Read the model definition and answer for the solid it produces. Units are mm, in the model's axes. Face numbers are marked on the shaded views. Coordinates: 2 decimals unless noted, no trailing zeros. Write each loop counter-clockwise with the first axis right and the second up, starting at its lowest first coordinate (ties: lowest second). Pieces come first, ordered by that corner, then holes. Notation, with made-up numbers: (-3, 87) -> (16, 87) arc R16 cw to (16, 102) -> close; hole circle Ø8 at (41, 26.5). An arc over 180 degrees is marked (long way). One line per item, written item: value. Start each with the question number.
1. Find section A-A, the plane x = 0. Write down the section's boundary in (y, z) (1 decimal).
2. Find section C-C, the plane x = -6.5. Write down the section's boundary in (y, z).
3. Find section D-D, the plane z = 12. Write down the section's boundary in (x, y) (3 decimals), and give its area (3 significant figures).
4. Consider line 1 along Z through (x, y) = (15, 0); line 2 along Y through (x, z) = (0, 26) (3 decimals); line 3 along X through (y, z) = (0.5, 23.5). Determine where each line is inside the solid, lowest interval first.
5. Given P1, Ø3, axis at x = -7.5, y = 7, coming from the -Z side; P2, Ø1.5, axis at y = -7, z = 28.5, coming from the +X side; P3, Ø8, axis at x = 10, z = 29.5, coming from the +Y side; P4, Ø6, axis at x = -6.5, z = 23.5, coming from the +Y side, each flat-ended and moving along its own axis, determine where each tip first touches the part or whether it passes through.
6. For a pull along Z with two mould halves and no side action, classify the marked faces 1, 2 and 3 as pulls with the +Z half, pulls with the -Z half, needs draft (parallel to the pull), parting line crosses it, or undercut.
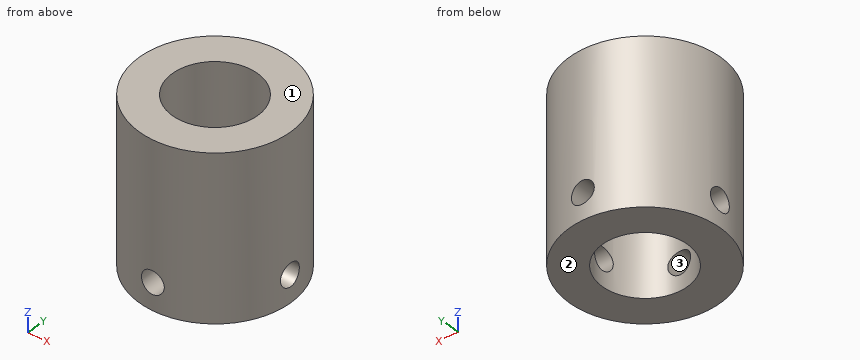
```python
from build123d import *

# Parameters (mm, degrees)
SKETCH1_R           = 16.891
SKETCH1_R_2         = 9.525
BOSS_EXTRUDE1_DEPTH = 36.5125
SKETCH2_R           = 2.54
CUT_EXTRUDE1_DEPTH  = 36.5125
CIRPATTERN1_COUNT   = 4


with BuildPart() as part:
    # Sketch1 → Boss-Extrude1 (new body)
    with BuildSketch(Plane.XY):
        Circle(SKETCH1_R)
        Circle(SKETCH1_R_2, mode=Mode.SUBTRACT)
    extrude(amount=BOSS_EXTRUDE1_DEPTH)

    # Sketch2 → Cut-Extrude1 (cut)
    with BuildSketch(Plane(origin=(16.891, 0, 0), x_dir=(0, 0, -1), z_dir=(1, 0, 0))):
        with Locations((-5.99948, 0)):
            Circle(SKETCH2_R)
    cut_extrude1 = extrude(amount=-CUT_EXTRUDE1_DEPTH, mode=Mode.SUBTRACT)

    # CirPattern1: Cut-Extrude1 ×4 about axis
    cirpattern1_axis = Axis((0, 0, 36.5125), (0, 0, -1))
    for i in range(1, CIRPATTERN1_COUNT):
        add(cut_extrude1.rotate(cirpattern1_axis, i * 360 / CIRPATTERN1_COUNT), mode=Mode.SUBTRACT)


solid = part.part
```
Answer block:
1. outline: (-16.9, 0) -> (-9.5, 0) -> (-9.5, 3.5) -> (-16.9, 3.5) -> close; (-16.9, 8.5) -> (-9.5, 8.5) -> (-9.5, 36.5) -> (-16.9, 36.5) -> close; (9.5, 0) -> (16.9, 0) -> (16.9, 3.5) -> (9.5, 3.5) -> close; (9.5, 8.5) -> (16.9, 8.5) -> (16.9, 36.5) -> (9.5, 36.5) -> close
2. outline: (-15.59, 0) -> (-6.96, 0) -> (-6.96, 36.51) -> (-15.59, 36.51) -> close; (6.96, 0) -> (15.59, 0) -> (15.59, 36.51) -> (6.96, 36.51) -> close
3. outline: circle Ø33.782 at (0, 0); hole circle Ø19.05 at (0, 0)
3. area: 611 mm2
4. line 1: z = 0 to 3.46, 8.54 to 36.51
4. line 2: y = -16.891 to -9.525, 9.525 to 16.891
4. line 3: x = -16.88 to -9.51, 9.51 to 16.88
5. P1: stops at z = 0
5. P2: stops at x = 15.69
5. P3: stops at y = 15.79
5. P4: stops at y = 16.52
6. face 1: pulls with the +Z half
6. face 2: pulls with the -Z half
6. face 3: undercut
